Could you check a few things on this model? Use its own coordinates, in mm. Face numbers are marked on the shaded views. A direction names the side the tool comes from. Give positions to 0.01 mm unless a question says otherwise; leave off trailing zeros. Write each loop counter-clockwise with the first axis right and the second up, starting at its lowest first coordinate (ties: lowest second). Pieces come first, ordered by that corner, then holes. Notation, with made-up numbers: (-10, 27.25) - (41, 27.25) arc R22 ccw to (41, 45.25) - close; hole circle Ø1 at (22, 23). An arc over 180 degrees is marked (long way). Answer as CSV lines item,"result". Start each with the question number.
Q1. We'd pull the mould along Z, two halves only. Please class the marked faces 1, 2 and 3: pulls with the +Z half, pulls with the -Z half, needs draft (parallel to the pull), parting line crosses it, or undercut.
Q2. Imagine slicing it at A-A on x = 0. List the corners of the cut face in (y, z) for me (3 decimals), and give its area (3 significant figures).
Q3. Imagine slicing it at B-B on z = 0. List the corners of the cut face in (x, y) for me (3 decimals).
Q4. Imagine slicing it at D-D on z = 32.5. List the corners of the cut face in (x, y) for me.
Q5. Will these pins go through, and if not, where does the flat tip stop? pin 1 Ø10.5 at (x, z) = (5, -1) entering from +Y; pin 2 Ø13.5 at (x, z) = (-7.5, 2) entering from +Y.
Q6. If I drill on line 1 along Z through (x, y) = (0, 58.2) (3 decimals); line 2 along Z through (x, y) = (0, 90.25), over which ranges is the centre line in solid material (lowest first)?
Q7. On a 3-axis mill with a long thin cutter (end or side, diameter ignored), from which of +Z, -Z, +X, -X, +Y, -Y can I reach the whole of each face in a straight line? I mean the marked faces 4, 5 and 6. Say none if no direction works.
Q8. Imagine slicing it at C-C on y = 67.5. List the corners of the cut face in (x, z) for me.
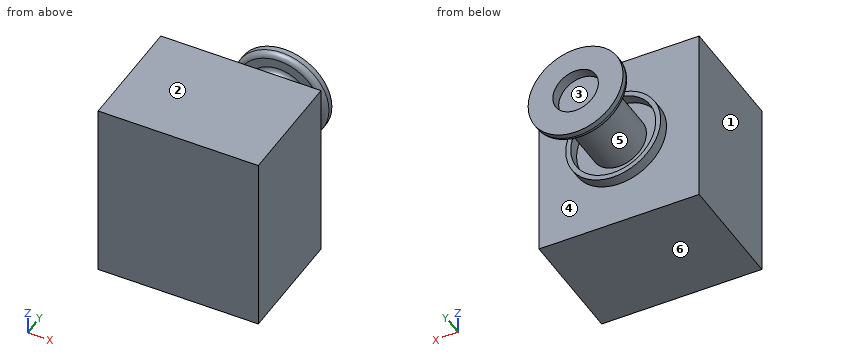
```python
from build123d import *

# Parameters (mm, degrees)
SKETCH1_W           = 75
SKETCH1_H           = 85
BOSS_EXTRUDE1_DEPTH = 55
SKETCH2_R           = 22.225
BOSS_EXTRUDE2_DEPTH = 5.08
SKETCH3_2_R         = 19.890557265
CUT_EXTRUDE1_DEPTH  = 5.08
SKETCH4_R           = 12.819708226
BOSS_EXTRUDE4_DEPTH = 33.02
SKETCH5_R           = 22.225
BOSS_EXTRUDE5_DEPTH = 5.08
FILLET1_R           = 2.54
SKETCH6_R           = 10.645057699
CUT_EXTRUDE2_DEPTH  = 5.08


with BuildPart() as part:
    # Sketch1 → Boss-Extrude1 (new body)
    with BuildSketch(Plane(origin=(0, 0, 0), x_dir=(1, 0, 0), z_dir=(0, 1, 0))):
        Rectangle(SKETCH1_W, SKETCH1_H)
    extrude(amount=BOSS_EXTRUDE1_DEPTH)

    # Sketch2 → Boss-Extrude2 (add)
    with BuildSketch(Plane(origin=(0, 55, 0), x_dir=(1, 0, 0), z_dir=(0, 1, 0))):
        Circle(SKETCH2_R)
    extrude(amount=BOSS_EXTRUDE2_DEPTH)

    # Sketch3<2> → Cut-Extrude1 (cut)
    with BuildSketch(Plane(origin=(0, 60.08, 0), x_dir=(1, 0, 0), z_dir=(0, 1, 0))):
        Circle(SKETCH3_2_R)
    extrude(amount=-CUT_EXTRUDE1_DEPTH, mode=Mode.SUBTRACT)

    # Sketch4 → Boss-Extrude4 (add)
    with BuildSketch(Plane(origin=(0, 55, 0), x_dir=(1, 0, 0), z_dir=(0, 1, 0))):
        Circle(SKETCH4_R)
    extrude(amount=BOSS_EXTRUDE4_DEPTH)

    # Sketch5 → Boss-Extrude5 (add)
    with BuildSketch(Plane(origin=(0, 88.02, 0), x_dir=(1, 0, 0), z_dir=(0, 1, 0))):
        Circle(SKETCH5_R)
    extrude(amount=BOSS_EXTRUDE5_DEPTH)

    # Fillet1
    fillet1_edges = [part.edges().sort_by_distance(p)[0] for p in [
        (-12.819708226, 88.02, 0),
        (-22.225, 88.02, 0),
    ]]
    fillet(fillet1_edges, radius=FILLET1_R)

    # Sketch6 → Cut-Extrude2 (cut)
    with BuildSketch(Plane(origin=(0, 93.1, 0), x_dir=(1, 0, 0), z_dir=(0, 1, 0))):
        Circle(SKETCH6_R)
    extrude(amount=-CUT_EXTRUDE2_DEPTH, mode=Mode.SUBTRACT)


solid = part.part
```
Conclusion:
1,face 1,"needs draft"
1,face 2,"pulls with the +Z half"
1,face 3,"undercut"
2,outline,"(0, -42.5) - (55, -42.5) - (55, -22.225) - (60.08, -22.225) - (60.08, -19.891) - (55, -19.891) - (55, -12.82) - (85.48, -12.82) arc R2.54 cw to (88.02, -15.36) - (88.02, -19.685) arc R2.54 ccw to (90.56, -22.225) - (93.1, -22.225) - (93.1, -10.645) - (88.02, -10.645) - (88.02, 10.645) - (93.1, 10.645) - (93.1, 22.225) - (90.56, 22.225) arc R2.54 ccw to (88.02, 19.685) - (88.02, 15.36) arc R2.54 cw to (85.48, 12.82) - (55, 12.82) - (55, 19.891) - (60.08, 19.891) - (60.08, 22.225) - (55, 22.225) - (55, 42.5) - (0, 42.5) - close"
2,area,"5,660 mm^2"
3,outline,"(-37.5, 0) - (37.5, 0) - (37.5, 55) - (22.225, 55) - (22.225, 60.08) - (19.891, 60.08) - (19.891, 55) - (12.82, 55) - (12.82, 85.48) arc R2.54 cw to (15.36, 88.02) - (19.685, 88.02) arc R2.54 ccw to (22.225, 90.56) - (22.225, 93.1) - (10.645, 93.1) - (10.645, 88.02) - (-10.645, 88.02) - (-10.645, 93.1) - (-22.225, 93.1) - (-22.225, 90.56) arc R2.54 ccw to (-19.685, 88.02) - (-15.36, 88.02) arc R2.54 cw to (-12.82, 85.48) - (-12.82, 55) - (-19.891, 55) - (-19.891, 60.08) - (-22.225, 60.08) - (-22.225, 55) - (-37.5, 55) - close"
4,outline,"(-37.5, 0) - (37.5, 0) - (37.5, 55) - (-37.5, 55) - close"
5,pin 1,"y = 88.02"
5,pin 2,"y = 93.1"
6,line 1,"-22.225 to -19.891, -12.82 to 12.82, 19.891 to 22.225"
6,line 2,"-22.21 to -10.65, 10.65 to 22.21"
7,face 4,"+Y"
7,face 5,"none"
7,face 6,"-Z, +X, -X, +Y, -Y"
8,outline,"circle Ø25.64 at (0, 0)"
